Build history of the part. All positions in model axes, mm. Face numbers are marked on the shaded views. A direction names the side the tool comes from. Coordinates: 2 decimals unless noted, no trailing zeros. Loops run counter-clockwise (first coordinate to the right, second up) from the corner with the lowest first, then second, coordinate; pieces in that order, holes last.
Item 1: Cut at D-D (z = 2). List the corners of the cut face in (x, y).
Item 2: Flat gauge pins, fed straight in: pin 1 (5 mm diameter, centred on x = -22.5, z = 9, fed in from +Y); pin 2 (1.8 mm diameter, centred on x = -27, z = 2.5, fed in from -Y); pin 3 (1 mm diameter, centred on y = -0.5, z = 4, fed in from -X); pin 4 (1.8 mm diameter, centred on x = 0, y = -10.29, fed in from +Z). Where does each tip first touch, or does it go through?
Item 3: Cut at B-B (x = -17). List the corners of the cut face in (y, z).
Item 4: 3-axis set-ups, long thin cutter, end or side, ignore diameter. For the marked faces 5, 6, 7 and 8: which of +Z, -Z, +X, -X, +Y, -Y reach the whole face in a straight line?
Item 5: Drill centre lines: line 1 along X through (y, z) = (0, 11); line 2 along Y through (x, z) = (-15, 1.5); line 3 along Y through (x, z) = (-10, 9). Where is each one in solid material? Low to high.
Item 6: Cut at C-C (x = 0). List the corners of the cut face in (y, z), and give its area (3 significant figures).
Item 7: Cut at A-A (y = 0). List the corners of the cut face in (x, z).
Item 8: Mould opens along Y. For the marked faces 1, 2, 3 and 4 say: released by +Y, released by -Y, zero draft, split by the parting line, or undercut.
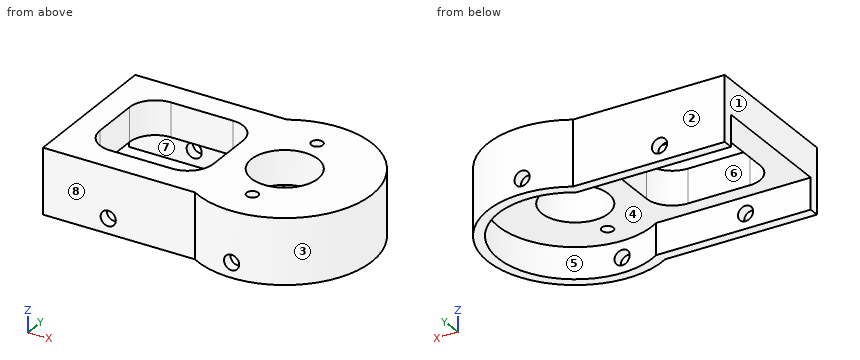
from build123d import *

# Parameters (mm, degrees)
SKETCH2_R           = 6.5
SKETCH2_R_2         = 1.1303
SKETCH2_W           = 22.1
SKETCH2_H           = 19.4
BOSS_EXTRUDE1_DEPTH = 12.7
CUT_EXTRUDE1_DEPTH  = 6.096
FILLET1_R           = 5
SKETCH6_R           = 1.4732
CUT_EXTRUDE4_DEPTH  = 53.620338273


with BuildPart() as part:
    # Sketch2 → Boss-Extrude1 (new body)
    with BuildSketch(Plane.XY):
        with BuildLine():
            Line((-38.1, -14.7), (-38.1, 14.7))
            Line((-38.1, 14.7), (-8.538735269, 14.7))
            ThreePointArc((-8.538735269, 14.7), (17, 0), (-8.538735269, -14.7))
            Line((-8.538735269, -14.7), (-38.1, -14.7))
        make_face()
        Circle(SKETCH2_R, mode=Mode.SUBTRACT)
        with Locations((0, -10.294657794)):
            Circle(SKETCH2_R_2, mode=Mode.SUBTRACT)
        with Locations((0, 10.294657794)):
            Circle(SKETCH2_R_2, mode=Mode.SUBTRACT)
        with Locations((-22.05, 0)):
            Rectangle(SKETCH2_W, SKETCH2_H, mode=Mode.SUBTRACT)
    extrude(amount=BOSS_EXTRUDE1_DEPTH)

    # Sketch1 → Cut-Extrude1 (cut)
    with BuildSketch(Plane.XY):
        with BuildLine():
            Line((-38.1, -12.7), (-38.1, 12.7))
            Line((-38.1, 12.7), (-7.981854421, 12.7))
            ThreePointArc((-7.981854421, 12.7), (15, 0), (-7.981854421, -12.7))
            Line((-7.981854421, -12.7), (-38.1, -12.7))
        make_face()
    extrude(amount=CUT_EXTRUDE1_DEPTH, mode=Mode.SUBTRACT)

    # Fillet1
    fillet1_edges = [part.edges().sort_by_distance(p)[0] for p in [
        (-33.1, 9.7, 9.398),
        (-33.1, -9.7, 9.398),
        (-11, -9.7, 9.398),
        (-11, 9.7, 9.398),
    ]]
    fillet(fillet1_edges, radius=FILLET1_R)

    # Sketch6 → Cut-Extrude4 (cut, through all)
    with BuildSketch(Plane(origin=(0, -17, 0), x_dir=(-1, 0, 0), z_dir=(0, -1, 0))):
        with Locations(Location((0, -2.921, 0), (0, 0, 180))):
            Circle(SKETCH6_R)
        with Locations(Location((25.4, -2.921, 0), (0, 0, 270))):
            Circle(SKETCH6_R)
    extrude(amount=-CUT_EXTRUDE4_DEPTH, mode=Mode.SUBTRACT)


solid = part.part
Filled sheet:
1. outline: (-38.1, -14.7) - (-26.55, -14.7) - (-26.55, -12.7) - (-38.1, -12.7) - close; (-38.1, 12.7) - (-26.55, 12.7) - (-26.55, 14.7) - (-38.1, 14.7) - close; (-24.25, -14.7) - (-8.54, -14.7) arc R17 ccw to (-1.15, -16.96) - (-1.15, -14.96) arc R15 cw to (-7.98, -12.7) - (-24.25, -12.7) - close; (-24.25, 12.7) - (-7.98, 12.7) arc R15 cw to (-1.15, 14.96) - (-1.15, 16.96) arc R17 ccw to (-8.54, 14.7) - (-24.25, 14.7) - close; (1.15, -16.96) arc R17 ccw to (1.15, 16.96) - (1.15, 14.96) arc R15 cw to (1.15, -14.96) - close
2. pin 1: stops at y = 14.7
2. pin 2: stops at y = -14.7
2. pin 3: stops at x = 14.97
2. pin 4: passes through
3. outline: (-14.7, 0) - (-12.7, 0) - (-12.7, 6.1) - (-9.7, 6.1) - (-9.7, 12.7) - (-14.7, 12.7) - close; (9.7, 6.1) - (12.7, 6.1) - (12.7, 0) - (14.7, 0) - (14.7, 12.7) - (9.7, 12.7) - close
4. face 5: -Z
4. face 6: +Z, -Z
4. face 7: -Z, -X
4. face 8: +Z, -Z, -X, -Y
5. line 1: x = -38.1 to -33.1, -11 to -6.5, 6.5 to 17
5. line 2: y = -14.7 to -12.7, 12.7 to 14.7
5. line 3: y = -14.7 to 14.7
6. outline: (-17, 0) - (-15, 0) - (-15, 1.45) - (-17, 1.45) - close; (-17, 4.39) - (-15, 4.39) - (-15, 6.1) - (-11.42, 6.1) - (-11.42, 12.7) - (-17, 12.7) - close; (-9.16, 6.1) - (-6.5, 6.1) - (-6.5, 12.7) - (-9.16, 12.7) - close; (6.5, 6.1) - (9.16, 6.1) - (9.16, 12.7) - (6.5, 12.7) - close; (11.42, 6.1) - (15, 6.1) - (15, 4.39) - (17, 4.39) - (17, 12.7) - (11.42, 12.7) - close; (15, 0) - (17, 0) - (17, 1.45) - (15, 1.45) - close
6. area: 121 mm2
7. outline: (-38.1, 6.1) - (-33.1, 6.1) - (-33.1, 12.7) - (-38.1, 12.7) - close; (-11, 6.1) - (-6.5, 6.1) - (-6.5, 12.7) - (-11, 12.7) - close; (6.5, 6.1) - (15, 6.1) - (15, 0) - (17, 0) - (17, 12.7) - (6.5, 12.7) - close
8. face 1: zero draft
8. face 2: released by +Y
8. face 3: split by the parting line
8. face 4: undercut
